```python
from build123d import *

# Parameters (mm, degrees)
SKETCH_1_W          = 210
SKETCH_1_H          = 70
EXTRUDE_1_DEPTH     = 4
SKETCH_2_R          = 1.65
CUT_EXTRUDE_1_DEPTH = 50
SKETCH_3_W          = 4
SKETCH_3_H          = 16
CUT_EXTRUDE_2_DEPTH = 50
FILLET_1_R          = 2
SKETCH_7_R          = 2.5
CUT_EXTRUDE_4_DEPTH = 100
SKETCH_8_R          = 12
CUT_EXTRUDE_5_DEPTH = 10
CUT_EXTRUDE_6_DEPTH = 10
SKETCH_10_R         = 2.5
CUT_EXTRUDE_7_DEPTH = 10


with BuildPart() as part:
    # 草图1 → 凸台-拉伸1 (new body)
    with BuildSketch(Plane(origin=(0, 0, 0), x_dir=(1, 0, 0), z_dir=(0, 1, 0))):
        Rectangle(SKETCH_1_W, SKETCH_1_H)
    extrude(amount=EXTRUDE_1_DEPTH)

    # 草图2 → 切除-拉伸1 (cut)
    with BuildSketch(Plane(origin=(0, 4, 0), x_dir=(1, 0, 0), z_dir=(0, 1, 0))):
        with Locations(Location((101, 19, 0), (0, 0, 270))):
            Circle(SKETCH_2_R)
        with Locations(Location((101, -19, 0), (0, 0, 270))):
            Circle(SKETCH_2_R)
        with Locations(Location((-101, -19, 0), (0, 0, 270))):
            Circle(SKETCH_2_R)
        with Locations(Location((-101, 19, 0), (0, 0, 270))):
            Circle(SKETCH_2_R)
        with Locations(Location((89, 19, 0), (0, 0, 270))):
            Circle(SKETCH_2_R)
        with Locations(Location((89, -19, 0), (0, 0, 270))):
            Circle(SKETCH_2_R)
        with Locations(Location((-89, -19, 0), (0, 0, 270))):
            Circle(SKETCH_2_R)
        with Locations(Location((-89, 19, 0), (0, 0, 270))):
            Circle(SKETCH_2_R)
    extrude(amount=-CUT_EXTRUDE_1_DEPTH, mode=Mode.SUBTRACT)

    # 草图3 → 切除-拉伸2 (cut)
    with BuildSketch(Plane(origin=(0, 4, 0), x_dir=(1, 0, 0), z_dir=(0, 1, 0))):
        with Locations((95, 0)):
            Rectangle(SKETCH_3_W, SKETCH_3_H)
        with Locations((-95, 0)):
            Rectangle(SKETCH_3_W, SKETCH_3_H)
    extrude(amount=-CUT_EXTRUDE_2_DEPTH, mode=Mode.SUBTRACT)

    # 圆角1
    fillet_1_edges = [part.edges().sort_by_distance(p)[0] for p in [
        (105, 2, 35),
        (-105, 2, 35),
        (-105, 2, -35),
        (105, 2, -35),
    ]]
    fillet(fillet_1_edges, radius=FILLET_1_R)

    # 草图7 → 切除-拉伸4 (cut)
    with BuildSketch(Plane(origin=(0, 4, 0), x_dir=(1, 0, 0), z_dir=(0, 1, 0))):
        with Locations(Location((27.223611076, 27.223611076, 0), (0, 0, 270))):
            Circle(SKETCH_7_R)
        with Locations(Location((-27.223611076, 27.223611076, 0), (0, 0, 270))):
            Circle(SKETCH_7_R)
        with Locations(Location((27.223611076, -27.223611076, 0), (0, 0, 270))):
            Circle(SKETCH_7_R)
        with Locations(Location((-27.223611076, -27.223611076, 0), (0, 0, 270))):
            Circle(SKETCH_7_R)
    extrude(amount=-CUT_EXTRUDE_4_DEPTH, mode=Mode.SUBTRACT)

    # 草图8 → 切除-拉伸5 (cut)
    with BuildSketch(Plane(origin=(0, 4, 0), x_dir=(1, 0, 0), z_dir=(0, 1, 0))):
        with Locations(Location((0, 0, 0), (0, 0, 270))):
            Circle(SKETCH_8_R)
    extrude(amount=-CUT_EXTRUDE_5_DEPTH, mode=Mode.SUBTRACT)

    # 草图9 → 切除-拉伸6 (cut)
    with BuildSketch(Plane(origin=(0, 4, 0), x_dir=(1, 0, 0), z_dir=(0, 1, 0))):
        with BuildLine():
            Line((27.5, 8), (72.5, 8))
            ThreePointArc((72.5, 8), (80.5, 0), (72.5, -8))
            Line((72.5, -8), (27.5, -8))
            ThreePointArc((27.5, -8), (19.5, 0), (27.5, 8))
        make_face()
        with BuildLine():
            Line((-27.5, 8), (-72.5, 8))
            ThreePointArc((-72.5, 8), (-80.5, 0), (-72.5, -8))
            Line((-72.5, -8), (-27.5, -8))
            ThreePointArc((-27.5, -8), (-19.5, 0), (-27.5, 8))
        make_face()
    extrude(amount=-CUT_EXTRUDE_6_DEPTH, mode=Mode.SUBTRACT)

    # 草图10 → 切除-拉伸7 (cut)
    with BuildSketch(Plane(origin=(0, 4, 0), x_dir=(1, 0, 0), z_dir=(0, 1, 0))):
        with Locations(Location((-90, -27.223611076, 0), (0, 0, 270))):
            Circle(SKETCH_10_R)
        with Locations(Location((-60, -27.223611076, 0), (0, 0, 270))):
            Circle(SKETCH_10_R)
        with Locations(Location((60, -27.223611076, 0), (0, 0, 270))):
            Circle(SKETCH_10_R)
        with Locations(Location((90, -27.223611076, 0), (0, 0, 270))):
            Circle(SKETCH_10_R)
        with Locations(Location((90, 27.223611076, 0), (0, 0, 270))):
            Circle(SKETCH_10_R)
        with Locations(Location((60, 27.223611076, 0), (0, 0, 270))):
            Circle(SKETCH_10_R)
        with Locations(Location((-60, 27.223611076, 0), (0, 0, 270))):
            Circle(SKETCH_10_R)
        with Locations(Location((-90, 27.223611076, 0), (0, 0, 270))):
            Circle(SKETCH_10_R)
    extrude(amount=-CUT_EXTRUDE_7_DEPTH, mode=Mode.SUBTRACT)


solid = part.part
```
Work out the finished part from the listing and answer in its coordinate system (mm). A direction names the side the tool comes from. Give positions to 0.01 mm unless a question says otherwise; leave off trailing zeros. Order: outer loops, then holes, each group sorted by start corner. A loop starts at its lowest first (then second) coordinate and runs counter-clockwise, first axis right, second up. Notation, with made-up numbers: (87.5, -32.75) - (126.5, -32.75) arc R24 cw to (126.5, -21.75) - close; hole circle Ø4 at (51.5, -23.5). An arc over 180 degrees is marked (long way). One line per item, written item: value. Start each with the question number.
1. Which of the six approach directions +Z, -Z, +X, -X, +Y, -Y give full straight-line access (tool end or side, diameter ignored) to faces 1 (the face through (-1, 0, -16)), 2 (the face through (50, 2, -8))?
2. Section B-B, the plane x = 60 is taken. Write down the section's boundary in (y, z).
3. Section D-D, the plane y = 2.95 is taken. Count the separate pieces of the cut face and the enclosed holes in it, then the cut area to 3 significant figures.
4. Section C-C, the plane z = 27 is taken. Write down the section's boundary in (x, y), then the cut area to 3 significant figures.
5. Consider line 1 (Z direction, x = 101, y = 3.15); line 2 (X direction, y = 2.15, z = 0); line 3 (X direction, y = 0.9, z = 19). Determine where each line is inside the solid, lowest interval first.
6. For a pull along Z with two mould halves and no side action, classify faces 3 (the face through (-1, 2, -35)), 4 (the face through (-1, 4, -16)), 5 (the face through (-1, 2, 35)), 6 (the face through (-95, 2, -8)) as released by +Z, released by -Z, zero draft, split by the parting line, or undercut.
7. Section A-A, the plane x = 0 is taken. Write down the section's boundary in (y, z), then the cut area to 3 significant figures.
Filled sheet:
1. face 1: +Z, -Z, +X, -X, -Y
1. face 2: +Y, -Y
2. outline: (0, -35) - (4, -35) - (4, -29.72) - (0, -29.72) - close; (0, -24.72) - (4, -24.72) - (4, -8) - (0, -8) - close; (0, 8) - (4, 8) - (4, 24.72) - (0, 24.72) - close; (0, 29.72) - (4, 29.72) - (4, 35) - (0, 35) - close
3. separate pieces: 1
3. enclosed holes: 25
3. area: 12,000 mm²
4. outline: (-105, 0) - (-92.49, 0) - (-92.49, 4) - (-105, 4) - close; (-87.51, 0) - (-62.49, 0) - (-62.49, 4) - (-87.51, 4) - close; (-57.51, 0) - (-29.71, 0) - (-29.71, 4) - (-57.51, 4) - close; (-24.73, 0) - (24.73, 0) - (24.73, 4) - (-24.73, 4) - close; (29.71, 0) - (57.51, 0) - (57.51, 4) - (29.71, 4) - close; (62.49, 0) - (87.51, 0) - (87.51, 4) - (62.49, 4) - close; (92.49, 0) - (105, 0) - (105, 4) - (92.49, 4) - close
4. area: 720 mm²
5. line 1: -35 to -20.65, -17.35 to 17.35, 20.65 to 35
5. line 2: -105 to -97, -93 to -80.5, -19.5 to -12, 12 to 19.5, 80.5 to 93, 97 to 105
5. line 3: -105 to -102.65, -99.35 to -90.65, -87.35 to 87.35, 90.65 to 99.35, 102.65 to 105
6. face 3: released by -Z
6. face 4: zero draft
6. face 5: released by +Z
6. face 6: undercut
7. outline: (0, -35) - (4, -35) - (4, -12) - (0, -12) - close; (0, 12) - (4, 12) - (4, 35) - (0, 35) - close
7. area: 184 mm²
